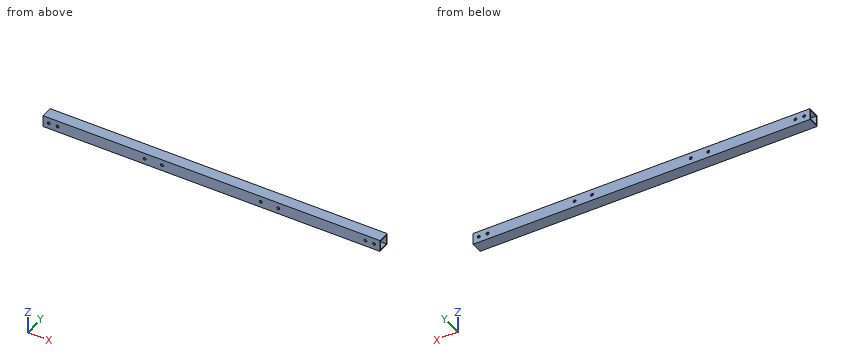
from build123d import *

# Parameters (mm, degrees)
SKETCH1_W           = 20
SKETCH1_H           = 20
SKETCH1_W_2         = 16
SKETCH1_H_2         = 16
BOSS_EXTRUDE1_DEPTH = 580
SKETCH2_R           = 2.5
CUT_EXTRUDE1_DEPTH  = 581.430874437
SKETCH3_R           = 2.5
CUT_EXTRUDE2_DEPTH  = 581.430874437


with BuildPart() as part:
    # Sketch1 → Boss-Extrude1 (new body)
    with BuildSketch(Plane(origin=(0, 0, 0), x_dir=(0, 0, -1), z_dir=(1, 0, 0))):
        Rectangle(SKETCH1_W, SKETCH1_H)
        Rectangle(SKETCH1_W_2, SKETCH1_H_2, mode=Mode.SUBTRACT)
    extrude(amount=BOSS_EXTRUDE1_DEPTH)

    # Sketch2 → Cut-Extrude1 (cut, through all)
    with BuildSketch(Plane(origin=(0, 10, 0), x_dir=(1, 0, 0), z_dir=(0, 1, 0))):
        with Locations(Location((10, 0, 0), (0, 0, 270))):
            Circle(SKETCH2_R)
        with Locations(Location((570, 0, 0), (0, 0, 270))):
            Circle(SKETCH2_R)
        with Locations(Location((25, 0, 0), (0, 0, 270))):
            Circle(SKETCH2_R)
        with Locations(Location((555, 0, 0), (0, 0, 270))):
            Circle(SKETCH2_R)
    extrude(amount=-CUT_EXTRUDE1_DEPTH, mode=Mode.SUBTRACT)

    # Sketch3 → Cut-Extrude2 (cut, through all)
    with BuildSketch(Plane(origin=(0, 10, 0), x_dir=(1, 0, 0), z_dir=(0, 1, 0))):
        with Locations(Location((175, 0, 0), (0, 0, 270))):
            Circle(SKETCH3_R)
        with Locations(Location((405, 0, 0), (0, 0, 270))):
            Circle(SKETCH3_R)
        with Locations(Location((205, 0, 0), (0, 0, 270))):
            Circle(SKETCH3_R)
        with Locations(Location((375, 0, 0), (0, 0, 270))):
            Circle(SKETCH3_R)
    extrude(amount=-CUT_EXTRUDE2_DEPTH, mode=Mode.SUBTRACT)


solid = part.part
Can you work these out from the model? Positions are in its coordinate system, mm. Round coordinates to 2 decimals unless told otherwise and drop trailing zeros. Order: outer loops, then holes, each group sorted by start corner. A loop starts at its lowest first (then second) coordinate and runs counter-clockwise, first axis right, second up. Notation, with made-up numbers: (-4.75, 86.5) - (21.25, 86.5) arc R24 ccw to (21.25, 118.5) - close; hole circle Ø5 at (-37.5, -28). An arc over 180 degrees is marked (long way). Answer in a Markdown table with one row per item.
(1) Suppose I cut it at B-B, the plane x = 290.5. Please give me the cut outline in (y, z).
From the geometry:
| item | result |
|---|---|
| outline | (-10, -10) - (10, -10) - (10, 10) - (-10, 10) - close; hole (-8, -8) - (8, -8) - (8, 8) - (-8, 8) - close |
(2) Please list where these lines run through material, in increasing order: L1, parallel to Z at x = 152, y = -2.75; L2, parallel to Z at x = 175, y = -9.4. Write a range as from..to.
From the geometry:
| item | result |
|---|---|
| L1 | z = -10..-8, 8..10 |
| L2 | z = -10..-2.5, 2.5..10 |
(3) For P1, Ø4, axis at x = 375, z = 0, coming from the -Y side, with a flat end and sliding along its axis, tell me the tip position at first contact or that it passes through.
From the geometry:
| item | result |
|---|---|
| P1 | passes through |
(4) Suppose I cut it at A-A, the plane y = -2.5. Please give me the cut outline in (x, z), plus the area to 3 significant figures.
From the geometry:
| item | result |
|---|---|
| outline | (0, -10) - (580, -10) - (580, -8) - (0, -8) - close; (0, 8) - (580, 8) - (580, 10) - (0, 10) - close |
| area | 2,320 mm2 |
